Design review of the part built by this model. Coordinates are the model's own, in mm. A direction names the side the tool comes from. Give positions to 0.01 mm unless a question says otherwise; leave off trailing zeros. Order: outer loops, then holes, each group sorted by start corner. A loop starts at its lowest first (then second) coordinate and runs counter-clockwise, first axis right, second up. Notation, with made-up numbers: (65, 84.25) -> (72, 84.25) arc R14 ccw to (72, 93.25) -> close; hole circle Ø9 at (-40, 7). An arc over 180 degrees is marked (long way). One line per item, written item: value. Start each with the question number.
1) The part is to be moulded in two halves that separate along Y. For faces 1 (the face through (-28.1, 7.43, 0.81)), 2 (the face through (-40.9, 49.43, 0.79)), 3 (the face through (-40.93, -49.4, 0.79)), say which applies: released by +Y, released by -Y, zero draft, split by the parting line, or undercut.
2) Wall thickness on line 1 along Y through (x, z) = (-39.5, 0.95); line 2 along X through (y, z) = (42.1, 1.1) (3 decimals); line 3 along X through (y, z) = (4.5, 1.4): over which ranges is each line inside the solid? List them lowest first. Write a range as from..to.
3) Tool access review of faces 4 (the face through (28.1, 7.43, 0.81)), 5 (the face through (40.93, 49.4, 0.79)): name each direction out of +Z, -Z, +X, -X, +Y, -Y from which nothing blocks a thin tool from reaching the whole face with its end or side.
4) Consider section B-B (z = 0.3). State how many separate pieces and enclosed holes the cut face has, plus the area to 3 significant figures.
5) For pin 1 (4 mm diameter, centred on x = 24.5, y = -10.5, fed in from -Z); pin 2 (1.3 mm diameter, centred on x = 39.5, y = -45, fed in from +Z), all flat-tipped, find the tip position at first contact; note any pin that passes through.
6) Consider section A-A (y = -45). State the section outline as (x, z) points.
from build123d import *

# Parameters (mm, degrees)
BOARDOUTLINE_DEPTH   = 1.6
SKETCH2_R            = 0.8
COMPONENTHOLES_DEPTH = 65.998538445
WINDOWS_1SIDE_DEPTH  = 65.998538445
M2_CLEARANCE_HOLE1_D = 2.1


with BuildPart() as part:
    # Sketch1 → boardOutline (new body)
    with BuildSketch(Plane.XY):
        with BuildLine():
            Line((-39.5, -50), (39.5, -50))
            ThreePointArc((39.5, -50), (40.914213562, -49.414213562), (41.5, -48))
            Line((41.5, -48), (41.5, 48))
            ThreePointArc((41.5, 48), (40.914213562, 49.414213562), (39.5, 50))
            Line((39.5, 50), (-39.5, 50))
            ThreePointArc((-39.5, 50), (-40.914213562, 49.414213562), (-41.5, 48))
            Line((-41.5, 48), (-41.5, -48))
            ThreePointArc((-41.5, -48), (-40.914213562, -49.414213562), (-39.5, -50))
        make_face()
    extrude(amount=BOARDOUTLINE_DEPTH)

    # Sketch2 → componentHoles (cut, through all)
    with BuildSketch(Plane.XY.offset(1.6)):
        with Locations((-5.385, 42.1)):
            Circle(SKETCH2_R)
        with Locations((5.385, 42.1)):
            Circle(SKETCH2_R)
    extrude(amount=-COMPONENTHOLES_DEPTH, mode=Mode.SUBTRACT)

    # Sketch3 → windows_1side (cut, through all)
    with BuildSketch(Plane.XY.offset(1.6)):
        with BuildLine():
            Line((37.5, -6), (37.5, 6))
            ThreePointArc((37.5, 6), (36.914213562, 7.414213562), (35.5, 8))
            Line((35.5, 8), (29.5, 8))
            ThreePointArc((29.5, 8), (28.085786438, 7.414213562), (27.5, 6))
            Line((27.5, 6), (27.5, -6))
            ThreePointArc((27.5, -6), (28.085786438, -7.414213562), (29.5, -8))
            Line((29.5, -8), (35.5, -8))
            ThreePointArc((35.5, -8), (36.914213562, -7.414213562), (37.5, -6))
        make_face()
        with BuildLine():
            Line((-29.5, -8), (-35.5, -8))
            ThreePointArc((-35.5, -8), (-36.914213562, -7.414213562), (-37.5, -6))
            Line((-37.5, -6), (-37.5, 6))
            ThreePointArc((-37.5, 6), (-36.914213562, 7.414213562), (-35.5, 8))
            Line((-35.5, 8), (-29.5, 8))
            ThreePointArc((-29.5, 8), (-28.085786438, 7.414213562), (-27.5, 6))
            Line((-27.5, 6), (-27.5, -6))
            ThreePointArc((-27.5, -6), (-28.085786438, -7.414213562), (-29.5, -8))
        make_face()
    extrude(amount=-WINDOWS_1SIDE_DEPTH, mode=Mode.SUBTRACT)

    # M2 Clearance Hole1 (through all)
    with Locations(Plane(origin=(0, 0, 0), x_dir=(-1, 0, 0), z_dir=(0, 0, -1))):
        with Locations((39.5, 45), (39.5, -15), (39.5, -45), (39.5, 15)):
            m2_clearance_hole1 = Hole(M2_CLEARANCE_HOLE1_D / 2)

    # Mirror1: M2 Clearance Hole1 across plane
    add(m2_clearance_hole1.mirror(Plane(origin=(0, 0, 0), x_dir=(0, 0, 1), z_dir=(1, 0, 0))), mode=Mode.SUBTRACT)


solid = part.part
Checked values:
1. face 1: undercut
1. face 2: released by +Y
1. face 3: released by -Y
2. line 1: y = -50..-46.05, -43.95..-16.05, -13.95..13.95, 16.05..43.95, 46.05..50
2. line 2: x = -41.5..-6.185, -4.585..4.585, 6.185..41.5
2. line 3: x = -41.5..-37.5, -27.5..27.5, 37.5..41.5
3. face 4: +Z, -Z
3. face 5: +Z, -Z, +X, +Y
4. separate pieces: 1
4. enclosed holes: 12
4. area: 7,950 mm^2
5. pin 1: stops at z = 0
5. pin 2: passes through
6. outline: (-41.5, 0) -> (-40.55, 0) -> (-40.55, 1.6) -> (-41.5, 1.6) -> close; (-38.45, 0) -> (38.45, 0) -> (38.45, 1.6) -> (-38.45, 1.6) -> close; (40.55, 0) -> (41.5, 0) -> (41.5, 1.6) -> (40.55, 1.6) -> close
